from build123d import *

# Parameters (mm, degrees)
F0_W        = 241.3
F0_H        = 38.1
F1_DEPTH    = 5.08
F2_W        = 241.3
F2_H        = 7.62
F3_DEPTH    = 10.16
F4_R        = 1.905
F5_DEPTH    = 22.861
F6_R        = 4.7625
F7_R        = 4.7625
F8_DEPTH    = 5.081
F9_T1_DEPTH = 251.46


# Not quite as in the source:
# - a fillet or chamfer that OpenCascade refuses, or shapes differently, is made with other operations: its cross-section is extruded or revolved along the edge and cut away or added


with BuildPart() as f1:
    # F0 (on Top) → F1 (new body)
    with BuildSketch(Plane.XY):
        with Locations((-10.1314700298, 19.05)):
            Rectangle(F0_W, F0_H)
    extrude(amount=F1_DEPTH)

    # F2 (on face) → F3 (join)
    with BuildSketch(Plane.XY.offset(5.08)):
        with Locations((-10.1314700298, 19.05)):
            Rectangle(F2_W, F2_H)
    extrude(amount=F3_DEPTH)

    # F4 (on face) → F5 (cut, through all)
    with BuildSketch(Plane.XZ.offset(-15.24)):
        with Locations((-119.3514700298, 11.43)):
            Circle(F4_R)
        with Locations((-106.6514700298, 11.43)):
            Circle(F4_R)
        with Locations((-93.9514700298, 11.43)):
            Circle(F4_R)
        with Locations((-81.2514700298, 11.43)):
            Circle(F4_R)
        with Locations((-68.5514700298, 11.43)):
            Circle(F4_R)
        with Locations((-55.8514700298, 11.43)):
            Circle(F4_R)
        with Locations((-43.1514700298, 11.43)):
            Circle(F4_R)
        with Locations((-30.4514700298, 11.43)):
            Circle(F4_R)
        with Locations((-17.7514700298, 11.43)):
            Circle(F4_R)
        with Locations((-5.0514700298, 11.43)):
            Circle(F4_R)
        with Locations((7.6485299702, 11.43)):
            Circle(F4_R)
        with Locations((20.3485299702, 11.43)):
            Circle(F4_R)
        with Locations((33.0485299702, 11.43)):
            Circle(F4_R)
        with Locations((45.7485299702, 11.43)):
            Circle(F4_R)
        with Locations((58.4485299702, 11.43)):
            Circle(F4_R)
        with Locations((71.1485299702, 11.43)):
            Circle(F4_R)
        with Locations((83.8485299702, 11.43)):
            Circle(F4_R)
        with Locations((96.5485299702, 11.43)):
            Circle(F4_R)
    extrude(amount=-F5_DEPTH, mode=Mode.SUBTRACT)

    # F6 (on face) + F7 (on face) → F8 (cut, through all)
    with BuildSketch(Plane.XY.offset(5.08)):
        with Locations((-114.719107688, 30.7975)):
            Circle(F6_R)
        with Locations((94.4530299702, 30.7975)):
            Circle(F6_R)
    with BuildSketch(Plane.XY.offset(5.08)):
        with Locations((-114.719107688, 7.3025)):
            Circle(F7_R)
        with Locations((94.4561676284, 7.3025)):
            Circle(F7_R)
    extrude(amount=-F8_DEPTH, mode=Mode.SUBTRACT)

    # F9: fillet of radius 2.032 on 2 edges, made by hand

    # F9_s2 → F9_t1 (cut)
    with BuildSketch(Plane.YZ.offset(-135.8614700298)):
        with BuildLine():
            ThreePointArc((15.24, 13.208), (15.8351590206, 14.6448409794), (17.272, 15.24))
            Line((17.272, 15.24), (15.24, 15.24))
            Line((15.24, 15.24), (15.24, 13.208))
        make_face()
        with BuildLine():
            ThreePointArc((20.828, 15.24), (22.2648409794, 14.6448409794), (22.86, 13.208))
            Line((22.86, 13.208), (22.86, 15.24))
            Line((22.86, 15.24), (20.828, 15.24))
        make_face()
    extrude(amount=F9_T1_DEPTH, mode=Mode.SUBTRACT)


solid = f1.part
CAD build for the part. Positions are in the model's coordinates, mm. A direction names the side the tool comes from. Coordinates: 2 decimals unless noted, no trailing zeros. Loops run counter-clockwise (first coordinate to the right, second up) from the corner with the lowest first, then second, coordinate; pieces in that order, holes last. Notation, with made-up numbers: (-40, 36.25) -> (-35, 36.25) arc R17 cw to (-35, 52.25) -> close; hole circle Ø3 at (73.5, -8). An arc over 180 degrees is marked (long way). One line per item, written item: value.
1. Pull direction Z, two halves, no side cores. Call faces 1 (the face through (-12, 31, 5.08)), 2 (the face through (-12, 22.86, 9)), 3 (the face through (81.945, 18.997, 11.514)): pulls with the +Z half, pulls with the -Z half, needs draft (parallel to the pull), parting line crosses it, or undercut.
Answers:
face 1: pulls with the +Z half
face 2: needs draft
face 3: undercut
2. Which spindle directions (+Z, -Z, +X, -X, +Y, -Y) get a long thin tool onto all of the face, cutting with end or side? Do faces 4 (the face through (-12, 15.24, 9)), 5 (the face through (-43.56, 19, 9.57)). Say none if no direction does.
Answers:
face 4: +Z, +X, -X, -Y
face 5: +Y, -Y
3. Drill centre lines: line 1 (X direction, y = 9, z = 4.75); line 2 (Y direction, x = -107, z = 9); line 3 (Z direction, x = 39, y = 23.5). Where is each one in solid material? Low to high. Write a range as [from, to].
Answers:
line 1: x = [-130.78, -119.17], [-110.27, 90.01], [98.91, 110.52]
line 2: y = [15.24, 22.86]
line 3: z = [0, 5.08]
4. Flat gauge pins, fed straight in: P1, Ø5, axis at x = 96.55, z = 11.43, coming from the -Y side; P2, Ø7.5, axis at x = -27, y = 11, coming from the +Z side; P3, Ø5, axis at x = -55.85, z = 11.43, coming from the +Y side. Where does each tip first touch, or does it go through?
Answers:
P1: stops at y = 15.24
P2: stops at z = 5.08
P3: stops at y = 22.86
5. Slice it at A-A on x = -24. Write the cut outline in (y, z), and give its area (3 significant figures).
Answers:
outline: (0, 0) -> (38.1, 0) -> (38.1, 5.08) -> (22.86, 5.08) -> (22.86, 13.21) arc R2.03 ccw to (20.83, 15.24) -> (17.27, 15.24) arc R2.03 ccw to (15.24, 13.21) -> (15.24, 5.08) -> (0, 5.08) -> close
area: 269 mm^2
